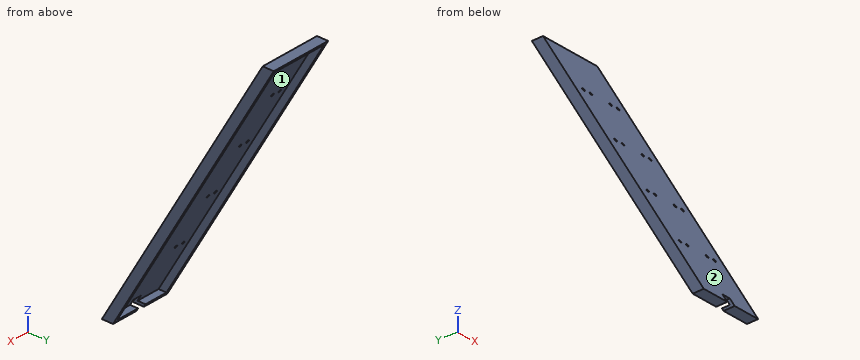
from build123d import *

# Parameters (mm, degrees)
BOSS_EXTRUDE1_DEPTH = 110
CUT_EXTRUDE1_DEPTH  = 100
SKETCH4_W           = 15
SKETCH4_H           = 30
CUT_EXTRUDE2_DEPTH  = 90
SKETCH7_R           = 2.5
CUT_EXTRUDE3_DEPTH  = 413


with BuildPart() as part:
    # Sketch1 → Boss-Extrude1 (new body)
    with BuildSketch(Plane(origin=(0, 0, 0), x_dir=(0, 0, -1), z_dir=(1, 0, 0))):
        Polygon((0, 20), (-500, 308.675134595), (-500, 288.675134595), (0, 0), align=None)
    extrude(amount=BOSS_EXTRUDE1_DEPTH)

    # Sketch3 → Cut-Extrude1 (cut)
    with BuildSketch(Plane(origin=(5, 0, 0), x_dir=(0, 0, -1), z_dir=(1, 0, 0))):
        Polygon((-495, 291.561885941), (-5, 8.660254038), (-5, 22.886751346), (-495, 305.788383249), align=None)
    extrude(amount=CUT_EXTRUDE1_DEPTH, mode=Mode.SUBTRACT)

    # Sketch4 → Cut-Extrude2 (cut)
    with BuildSketch(Plane(origin=(0, 0, 0), x_dir=(1, 0, 0), z_dir=(0, 1, 0))):
        with Locations((55, 0)):
            Rectangle(SKETCH4_W, SKETCH4_H)
    extrude(amount=CUT_EXTRUDE2_DEPTH, mode=Mode.SUBTRACT)

    # Sketch7 → Cut-Extrude3 (cut)
    with BuildSketch(Plane(origin=(0, 0, 0), x_dir=(1, 0, 0), z_dir=(0, 1, 0))):
        with Locations((20, -105)):
            Circle(SKETCH7_R)
        with Locations((90, -105)):
            Circle(SKETCH7_R)
        with Locations((20, -205)):
            Circle(SKETCH7_R)
        with Locations((20, -305)):
            Circle(SKETCH7_R)
        with Locations((20, -405)):
            Circle(SKETCH7_R)
        with Locations((35, -205)):
            Circle(SKETCH7_R)
        with Locations((35, -305)):
            Circle(SKETCH7_R)
        with Locations((35, -405)):
            Circle(SKETCH7_R)
        with Locations((35, -105)):
            Circle(SKETCH7_R)
        with Locations((90, -205)):
            Circle(SKETCH7_R)
        with Locations((90, -305)):
            Circle(SKETCH7_R)
        with Locations((90, -405)):
            Circle(SKETCH7_R)
        with Locations((75, -205)):
            Circle(SKETCH7_R)
        with Locations((75, -305)):
            Circle(SKETCH7_R)
        with Locations((75, -405)):
            Circle(SKETCH7_R)
        with Locations((75, -105)):
            Circle(SKETCH7_R)
    extrude(amount=CUT_EXTRUDE3_DEPTH, mode=Mode.SUBTRACT)


solid = part.part
Geometry: final body of the model. Coordinates: model frame, mm. Face numbers are marked on the shaded views. Give positions to 0.01 mm unless a question says otherwise; leave off trailing zeros. Write each loop counter-clockwise with the first axis right and the second up, starting at its lowest first coordinate (ties: lowest second). Pieces come first, ordered by that corner, then holes. Notation, with made-up numbers: (59, 47.25) -> (85, 47.25) arc R29 ccw to (85, 68.25) -> close; hole circle Ø4 at (-1.75, 88). An arc over 180 degrees is marked (long way). Answer in a Markdown table with one row per item.
(1) Section query B-B on y = 269. Return loops of the section in (x, z).
Answers below:
| item | result |
|---|---|
| outline | (0, 431.28) -> (5, 431.28) -> (5, 455.92) -> (105, 455.92) -> (105, 431.28) -> (110, 431.28) -> (110, 465.92) -> (0, 465.92) -> close |
(2) Section query A-A on z = 387. Return loops of the section in (x, y), then the cut area to 3 significant figures.
Answers below:
| item | result |
|---|---|
| outline | (0, 223.43) -> (110, 223.43) -> (110, 243.43) -> (105, 243.43) -> (105, 229.21) -> (5, 229.21) -> (5, 243.43) -> (0, 243.43) -> close |
| area | 777 mm^2 |
(3) Draft query along X for the marked faces 1 and 2. Return one class per face: +X half, -X half, draft (parallel to the pull), parting line (faces both ways), or undercut.
Answers below:
| item | result |
|---|---|
| face 1 | undercut |
| face 2 | draft |
(4) Pin query (flat end, axial travel): pin 1 (3 mm diameter, centred on x = 75, z = 205, fed in from -Y); pin 2 (3 mm diameter, centred on x = 28, y = 43, fed in from +Z); pin 3 (6 mm diameter, centred on x = 73, z = 288, fed in from +Y); pin 4 (1.7 mm diameter, centred on x = 54, y = 12.5, fed in from -Z). Return the tip coordinate at first contact, or that it passes through.
Answers below:
| item | result |
|---|---|
| pin 1 | through |
| pin 2 | z = 77.08 |
| pin 3 | y = 173.78 |
| pin 4 | z = 15 |
(5) Ray query, line 1 along X through (y, z) = (122, 205); line 2 along X through (y, z) = (141, 233); line 3 along Y through (x, z) = (88, 299). Return the intervals inside material, ascending. Write a range as [from, to].
Answers below:
| item | result |
|---|---|
| line 1 | [0, 17.5], [22.5, 32.5], [37.5, 72.5], [77.5, 87.5], [92.5, 110] |
| line 2 | [0, 5], [105, 110] |
| line 3 | [172.63, 178.4] |
